For this review, use the dimensioned drawing (mm, ordinates from the lowest corner) and the shaded views. A direction names the side the tool comes from. Coordinates: 2 decimals unless noted, no trailing zeros. Write each loop counter-clockwise with the first axis right and the second up, starting at its lowest first coordinate (ties: lowest second). Pieces come first, ordered by that corner, then holes. Notation, with made-up numbers: (66.25, 54.25) -> (117.25, 54.25) arc R17 cw to (117.25, 81.25) -> close; hole circle Ø7 at (74.5, -17). An arc over 180 degrees is marked (long way). Put each result on its own line as item: value. Start each with the question number.
Item 1: To check wall thickness, follow L1, parallel to X at y = 2.5, z = 6.5; L2, parallel to X at y = 4.25, z = 4.75 (1 decimal); L3, parallel to Y at x = 3.4, z = 4.5 (1 decimal). State the ranges of each line that lie inside material, in increasing order.
Item 2: Consider section A-A on z = 19.25. Give the boundary of the cut face in (x, y), and give its area (3 significant figures).
Item 3: The part is to be moulded in two halves that separate along Y. For the marked faces 3, 4 and 5, say which applies: +Y half, -Y half, draft (parallel to the pull), parting line (faces both ways), or undercut.
Item 4: Consider section D-D on y = 5.5. Give the boundary of the cut face in (x, z).
Item 5: Insertion check: P1, Ø2, axis at x = 2.75, y = 3.18, coming from the +Z side; P2, Ø1, axis at y = 1, z = 14.5, coming from the -X side. Each pin has a flat end and moves straight along its axis. Give the tip position at first contact, or say it passes through.
Item 6: For the marked faces 1 and 2, list the 3-axis set-ups (+Z, -Z, +X, -X, +Y, -Y) from which the entire face can be reached by the end or side of a thin tool; tool diameter is ignored.
Item 7: Consider section C-C on x = 0.5. Give the boundary of the cut face in (y, z).
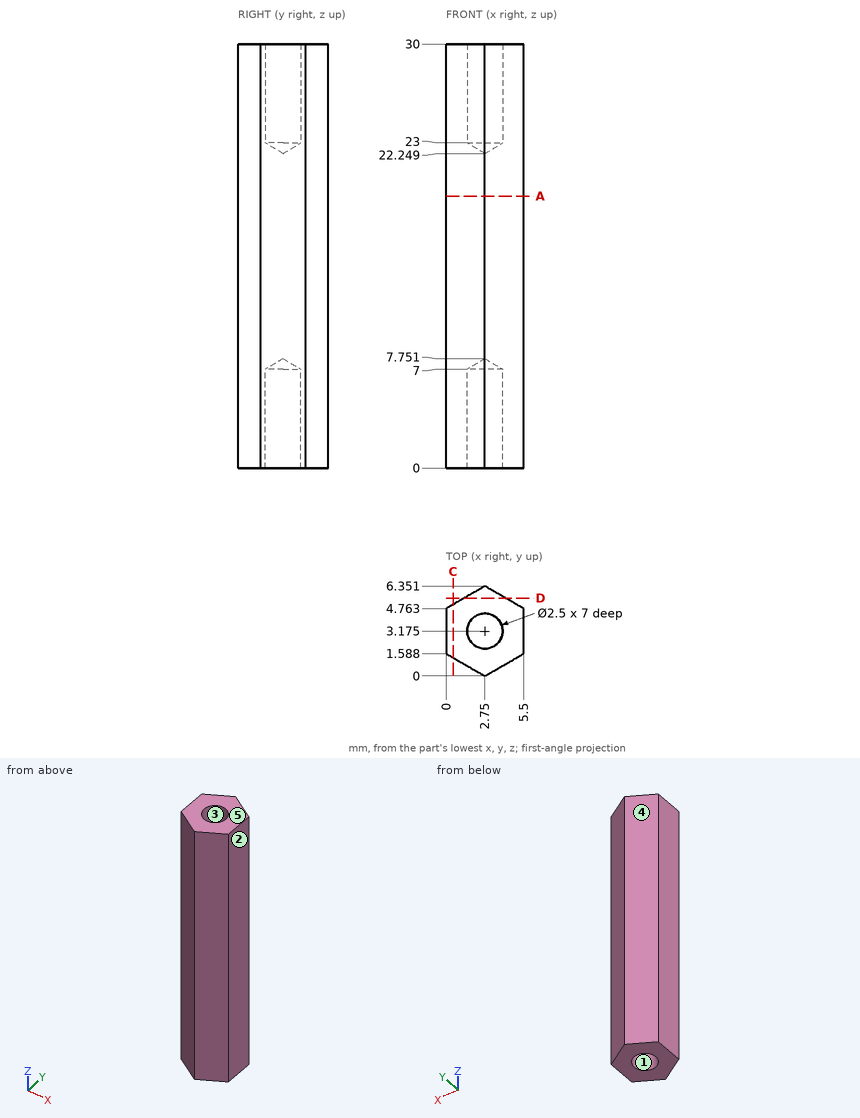
Return value:
1. L1: 0 to 1.7, 3.8 to 5.5
1. L2: 0 to 2.1, 3.4 to 5.5
1. L3: 0.4 to 2.1, 4.2 to 6
2. outline: (0, 1.59) -> (2.75, 0) -> (5.5, 1.59) -> (5.5, 4.76) -> (2.75, 6.35) -> (0, 4.76) -> close
2. area: 26.2 mm^2
3. face 3: undercut
3. face 4: +Y half
3. face 5: draft
4. outline: (1.28, 0) -> (4.22, 0) -> (4.22, 30) -> (1.28, 30) -> close
5. P1: z = 22.85
5. P2: x = 0.15
6. face 1: -Z
6. face 2: +Z, -Z, +X, +Y, -Y
7. outline: (1.3, 0) -> (5.05, 0) -> (5.05, 30) -> (1.3, 30) -> close
